The listing builds one solid part. Answer for the finished solid, in the listing's coordinates (mm). A direction names the side the tool comes from. Round coordinates to 2 decimals unless told otherwise and drop trailing zeros. Loops run counter-clockwise (first coordinate to the right, second up) from the corner with the lowest first, then second, coordinate; pieces in that order, holes last. Notation, with made-up numbers: M 24.5,64 L 46.5,64 A12 ccw 46.5,69 Z; hole C -27,31.25 d6. An arc over 180 degrees is marked long. Answer as a JSON object with one key per item and string values.
```python
from build123d import *

# Parameters (mm, degrees)
SKETCH1_R               = 14.2875
SKETCH1_R_2             = 3.2639
SKETCH1_R_3             = 2.4892
BOSS_EXTRUDE1_DEPTH     = 4.7625
CUT_EXTRUDE1_DEPTH      = 446.923725363
CUT_EXTRUDE1_DEPTH_BACK = 446.923725363
SKETCH2_R               = 19.685
SKETCH2_R_2             = 2.4892
SKETCH2_R_3             = 3.175
FILLET3_R               = 38.1
FILLET4_R               = 10.16


with BuildPart() as part:
    # Sketch1 → Boss-Extrude1 (new body)
    with BuildSketch(Plane.XY):
        with BuildLine():
            Line((27.94, 38.1), (164.412883856, 38.1))
            Line((164.412883856, 38.1), (299.654886368, -56.597469642))
            Line((299.654886368, -56.597469642), (352.6409093, 76.843527732))
            Line((352.6409093, 76.843527732), (368.245755744, 65.91689662))
            Line((368.245755744, 65.91689662), (359.391134552, -13.154135899))
            Line((359.391134552, -13.154135899), (424.411328067, -58.681765534))
            ThreePointArc((424.411328067, -58.681765534), (428.328306358, -64.830189864), (426.750435733, -71.947504312))
            Line((426.750435733, -71.947504312), (393.970542395, -118.762043644))
            ThreePointArc((393.970542395, -118.762043644), (387.822118066, -122.679021935), (380.704803617, -121.101151309))
            Line((380.704803617, -121.101151309), (346.894302989, -97.426783899))
            Line((346.894302989, -97.426783899), (328.683251135, -123.434861305))
            Line((328.683251135, -123.434861305), (152.4, 0))
            Line((152.4, 0), (51.495079847, 0))
            ThreePointArc((51.495079847, 0), (37.452913318, 1.305023138), (23.891727162, 5.175392148))
            Line((23.891727162, 5.175392148), (22.419329463, 5.747632027))
            ThreePointArc((22.419329463, 5.747632027), (15.362388562, 11.346666629), (12.7, 19.952553597))
            Line((12.7, 19.952553597), (12.7, 22.86))
            ThreePointArc((12.7, 22.86), (17.163692655, 33.636307345), (27.94, 38.1))
        make_face()
        with Locations(Location((324.005035804, -96.903383749, 0), (0, 0, 180))):
            Circle(SKETCH1_R, mode=Mode.SUBTRACT)
        with Locations(Location((347.013016961, 7.916185169, 0), (0, 0, 180))):
            Circle(SKETCH1_R_2, mode=Mode.SUBTRACT)
        with Locations(Location((324.005035804, -77.853383749, 0), (0, 0, 180))):
            Circle(SKETCH1_R_3, mode=Mode.SUBTRACT)
        with Locations(Location((355.344238002, 64.097950502, 0), (0, 0, 180))):
            Circle(SKETCH1_R_2, mode=Mode.SUBTRACT)
        with Locations(Location((391.63143473, -105.496304865, 0), (0, 0, 180))):
            Circle(SKETCH1_R_2, mode=Mode.SUBTRACT)
        with Locations(Location((266.78726551, -56.83906967, 0), (0, 0, 180))):
            Circle(SKETCH1_R_2, mode=Mode.SUBTRACT)
        Polygon((18.067651581, 19.05), (21.733825791, 12.7), (29.066174209, 12.7), (32.732348419, 19.05), (29.066174209, 25.4), (21.733825791, 25.4), align=None, mode=Mode.SUBTRACT)
    extrude(amount=BOSS_EXTRUDE1_DEPTH)

    # Sketch2 → Cut-Extrude1 (cut, two sides: drawn at the far end of the back side and taken through both)
    with BuildSketch(Plane.XY.offset(4.7625).offset(-CUT_EXTRUDE1_DEPTH_BACK)):
        with Locations((382.793006548, -68.299896272)):
            Circle(SKETCH2_R)
        with Locations((395.493006548, -90.296941528)):
            Circle(SKETCH2_R_2)
        with Locations((360.795961291, -80.999896272)):
            Circle(SKETCH2_R_2)
        with Locations((370.093006548, -46.302851016)):
            Circle(SKETCH2_R_2)
        with Locations((404.790051804, -55.599896272)):
            Circle(SKETCH2_R_2)
        with Locations((179.07, -10.598705626)):
            Circle(SKETCH2_R_3)
    extrude(amount=CUT_EXTRUDE1_DEPTH + CUT_EXTRUDE1_DEPTH_BACK, mode=Mode.SUBTRACT)

    # Fillet3
    fillet3_edges = [part.edges().sort_by_distance(p)[0] for p in [
        (164.412883856, 38.1, 2.38125),
        (299.654886368, -56.597469642, 2.38125),
        (359.391134552, -13.154135899, 2.38125),
        (152.4, 0, 2.38125),
    ]]
    fillet(fillet3_edges, radius=FILLET3_R)

    # Fillet4
    fillet4_edges = [part.edges().sort_by_distance(p)[0] for p in [
        (352.6409093, 76.843527732, 2.38125),
        (368.245755744, 65.91689662, 2.38125),
        (346.894302989, -97.426783899, 2.38125),
        (328.683251135, -123.434861305, 2.38125),
    ]]
    fillet(fillet4_edges, radius=FILLET4_R)


solid = part.part
```
Item 1: The part is cut by section A-A (x = 55.5). Give the vertices of the cut face in (y, z), then the cut area to 3 significant figures.
Values follow:
{"outline": "M 0,0 L 38.1,0 L 38.1,4.76 L 0,4.76 Z", "area": "181 mm^2"}
Item 2: The part is cut by section C-C (y = 50). Give the vertices of the cut face in (x, z).
Values follow:
{"outline": "M 341.98,0 L 366.46,0 L 366.46,4.76 L 341.98,4.76 Z"}
Item 3: Which of the six approach directions +Z, -Z, +X, -X, +Y, -Y give full straight-line access (tool end or side, diameter ignored) to faces 4 (the face through (368.139, -112.303, 2.348)), 5 (the face through (400.839, -42.176, 2.348)), 6 (the face through (163.701, 36.385, 2.415))?
Values follow:
{"face 4": "+Z, -Z, -Y", "face 5": "+Z, -Z, +X, +Y", "face 6": "+Z, -Z, +Y"}
Item 4: Determine the mould class of faces 1 (the face through (364.932, -10.338, 2.415)), 2 (the face through (292.5, -34.38, 2.41)), 3 (the face through (15.435, 11.241, 2.348)) for opening direction X: released by +X, released by -X, zero draft, split by the parting line, or undercut.
Values follow:
{"face 1": "released by +X", "face 2": "undercut", "face 3": "released by -X"}
Item 5: The part is cut by section B-B (z = 3.6). Give the number of separate pieces and of enclosed holes in the cut face, then the cut area to 3 significant figures.
Values follow:
{"separate pieces": "1", "enclosed holes": "13", "area": "22,900 mm^2"}
Item 6: Straight lines are drawn through the part: line 1 (X direction, y = -8, z = 0.55); line 2 (X direction, y = -56, z = 0.55); line 3 (X direction, y = -11, z = 2.35). For each, find the intervals that lie inside material, in ascending order.
Values follow:
{"line 1": "163.83 to 177.25, 180.89 to 230.25, 318.95 to 363.99", "line 2": "232.38 to 263.63, 269.94 to 367.42, 398.16 to 402.33, 407.25 to 420.58", "line 3": "168.11 to 175.92, 182.22 to 234.53, 317.76 to 365.23"}
Item 7: Flat-ended cylindrical pins translate along their axes: P1, Ø2.5, axis at x = 26.5, z = 3.5, coming from the +Y side; P2, Ø1.4, axis at x = 26, z = 1.5, coming from the -Y side; P3, Ø1, axis at x = 119.5, z = 3.5, coming from the -Y side. Find the tip coordinate at first contact, or state that the pin passes through.
Values follow:
{"P1": "y = 38.1", "P2": "y = 4.15", "P3": "y = 0"}
